```python
from build123d import *

# Parameters (mm, degrees)
SKETCH1_W                                       = 56
SKETCH1_H                                       = 10
BOSS_EXTRUDE1_DEPTH                             = 10
CSK_FOR_M3_FLAT_HEAD_MACHINE_SCREW1_D           = 3.4
CSK_FOR_M3_FLAT_HEAD_MACHINE_SCREW1_CSINK_D     = 6.3
CSK_FOR_M3_FLAT_HEAD_MACHINE_SCREW1_CSINK_ANGLE = 90
F_5_0MM_DOWEL_HOLE1_D                           = 5
F_5_0MM_DOWEL_HOLE1_DEPTH                       = 5
F_5_0MM_DOWEL_HOLE1_TIP                         = 1.502151548


with BuildPart() as part:
    # Sketch1 → Boss-Extrude1 (new body)
    with BuildSketch(Plane(origin=(0, 0, 0), x_dir=(1, 0, 0), z_dir=(0, 1, 0))):
        with Locations((0.542682927, 11.422256098)):
            Rectangle(SKETCH1_W, SKETCH1_H)
    extrude(amount=BOSS_EXTRUDE1_DEPTH)

    # CSK for M3 Flat Head Machine Screw1 (through all)
    with Locations(Plane(origin=(0, 10, 0), x_dir=(1, 0, 0), z_dir=(0, 1, 0))):
        with Locations((15.042682927, 11.422256098), (-13.957317073, 11.422256098)):
            CounterSinkHole(CSK_FOR_M3_FLAT_HEAD_MACHINE_SCREW1_D / 2, CSK_FOR_M3_FLAT_HEAD_MACHINE_SCREW1_CSINK_D / 2, counter_sink_angle=CSK_FOR_M3_FLAT_HEAD_MACHINE_SCREW1_CSINK_ANGLE)

    # Ø5.0mm Dowel Hole1
    with Locations(Plane(origin=(0, 0, 0), x_dir=(-1, 0, 0), z_dir=(0, -1, 0))):
        with Locations((22.457317073, 11.422256098), (-23.542682927, 11.422256098)):
            Hole(F_5_0MM_DOWEL_HOLE1_D / 2, depth=F_5_0MM_DOWEL_HOLE1_DEPTH)
            with Locations((0, 0, -(F_5_0MM_DOWEL_HOLE1_DEPTH + F_5_0MM_DOWEL_HOLE1_TIP / 2))):  # 118° drill point
                Cone(0, F_5_0MM_DOWEL_HOLE1_D / 2, F_5_0MM_DOWEL_HOLE1_TIP, mode=Mode.SUBTRACT)


solid = part.part
```
The listing builds one solid part. Answer for the finished solid, in the listing's coordinates (mm). A direction names the side the tool comes from. Give positions to 0.01 mm unless a question says otherwise; leave off trailing zeros. Order: outer loops, then holes, each group sorted by start corner. A loop starts at its lowest first (then second) coordinate and runs counter-clockwise, first axis right, second up.
1) Consider line 1 along X through (y, z) = (1.25, -10.5); line 2 along X through (y, z) = (9.75, -11.25); line 3 along X through (y, z) = (2, -10.25). Determine where each line is inside the solid, lowest interval first.
Reported:
line 1: x = -27.46 to -24.78, -20.13 to -15.39, -12.53 to 13.61, 16.47 to 21.22, 25.87 to 28.54
line 2: x = -27.46 to -16.85, -11.06 to 12.15, 17.94 to 28.54
line 3: x = -27.46 to -24.67, -20.25 to -15.19, -12.73 to 13.81, 16.27 to 21.33, 25.75 to 28.54
2) Find section A-A on y = 7.25. Write down the section's boundary in (x, z).
Reported:
outline: (-27.46, -16.42) - (28.54, -16.42) - (28.54, -6.42) - (-27.46, -6.42) - close; hole circle Ø3.4 at (-13.96, -11.42); hole circle Ø3.4 at (15.04, -11.42)
3) Determine the mould class of faces 3 (the face through (0, 10, -11)), 4 (the face through (23.89, 6.24, -11.16)), 5 (the face through (-15.528, 4.215, -10.771)), 6 (the face through (0, 5, -16.422)) for opening direction Z: pulls with the +Z half, pulls with the -Z half, needs draft (parallel to the pull), parting line crosses it, or undercut.
Reported:
face 3: needs draft
face 4: undercut
face 5: undercut
face 6: pulls with the -Z half
4) Find section C-C on z = -12.25. Give the number of separate pieces and of enclosed holes in the cut face, then the cut area to 3 significant figures.
Reported:
separate pieces: 3
enclosed holes: 0
area: 443 mm2
5) For faces 1 (the face through (0, 5, -6.422)), 2 (the face through (-21.11, 2.54, -13.53)), determine the directions among +Z, -Z, +X, -X, +Y, -Y from which every point of the face is accessible in a straight line to the end or side of a thin tool.
Reported:
face 1: +Z, +X, -X, +Y, -Y
face 2: -Y
6) Given P1, Ø2, axis at x = -13.96, z = -11.42, coming from the -Y side; P2, Ø4.5, axis at x = 23.54, z = -11.42, coming from the -Y side, each flat-ended and moving along its own axis, determine where each tip first touches the part or whether it passes through.
Reported:
P1: passes through
P2: stops at y = 5.15
7) Find section B-B on y = 2. Write down the section's boundary in (x, z), then the cut area to 3 significant figures.
Reported:
outline: (-27.46, -16.42) - (28.54, -16.42) - (28.54, -6.42) - (-27.46, -6.42) - close; hole circle Ø5 at (-22.46, -11.42); hole circle Ø3.4 at (-13.96, -11.42); hole circle Ø3.4 at (15.04, -11.42); hole circle Ø5 at (23.54, -11.42)
area: 503 mm2
